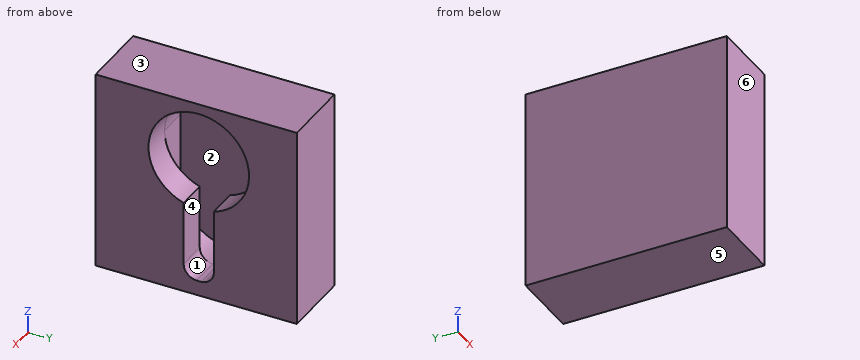
from build123d import *

# Parameters (mm, degrees)
F0_W     = 7
F0_H     = 20
F1_DEPTH = 20
F3_DEPTH = 6
F4_W     = 36.7105286568
F4_H     = 22.0389235765
F5_DEPTH = 3
F6_W     = 20
F6_H     = 20
F7_DEPTH = 3


# Not quite as in the source:
# - after a boolean that leaves OpenCascade's solid faulty, fix() repairs it


with BuildPart() as f1:
    # F0 (on Top) → F1 (new body)
    with BuildSketch(Plane.XY):
        with Locations((-6.9235885665, -0.25)):
            Rectangle(F0_W, F0_H)
    extrude(amount=F1_DEPTH)

    # F2 (on face) → F3 (cut)
    with BuildSketch(Plane.YZ.offset(-3.4235885665)):
        with BuildLine():
            Line((5, 6.5), (5, 14))
            ThreePointArc((5, 14), (0, 19), (-5, 14))
            Line((-5, 14), (-5, 6.5))
            ThreePointArc((-5, 6.5), (-3.5355339059, 2.9644660941), (0, 1.5))
            ThreePointArc((0, 1.5), (3.5355339059, 2.9644660941), (5, 6.5))
        make_face()
    extrude(amount=-F3_DEPTH, mode=Mode.SUBTRACT)

    # F4 (on face) → F5 (cut)
    with BuildSketch(Plane.YZ.offset(-3.4235885665)):
        with Locations((-1.3269511983, 11.0194617882)):
            Rectangle(F4_W, F4_H)
    extrude(amount=-F5_DEPTH, mode=Mode.SUBTRACT)

    # F6 (on face) → F7 (join)
    with BuildSketch(Plane.YZ.offset(-6.4235885665)):
        with Locations((-0.25, 10)):
            Rectangle(F6_W, F6_H)
        with BuildLine():
            ThreePointArc((-1.5, 9.2303039929), (0, 19), (1.5, 9.2303039929))
            Line((1.5, 9.2303039929), (1.5, 2.8392676962))
            ThreePointArc((1.5, 2.8392676962), (1.1297736268, 1.9163028593), (0.2243504639, 1.505035849))
            ThreePointArc((0.2243504639, 1.505035849), (0, 1.5), (-0.2243504639, 1.505035849))
            ThreePointArc((-0.2243504639, 1.505035849), (-1.1297736268, 1.9163028593), (-1.5, 2.8392676962))
            Line((-1.5, 2.8392676962), (-1.5, 9.2303039929))
        make_face(mode=Mode.SUBTRACT)
    extrude(amount=F7_DEPTH)

    add(f1.part.fix(), mode=Mode.REPLACE)


solid = f1.part
Model file for the job. Use its own axes, mm. Face numbers are marked on the shaded views. A direction names the side the tool comes from. Give positions to 0.01 mm unless a question says otherwise; leave off trailing zeros. Loops run counter-clockwise (first coordinate to the right, second up) from the corner with the lowest first, then second, coordinate; pieces in that order, holes last. Notation, with made-up numbers: (-1, -8) - (42, -8) arc R29 cw to (42, 29) - close; hole circle Ø5 at (80, -4). An arc over 180 degrees is marked (long way). Use one line per item in the form item = value.
(1) Pull direction Y, two halves, no side cores. Call the marked faces 4, 5 and 6: pulls with the +Y half, pulls with the -Y half, needs draft (parallel to the pull), parting line crosses it, or undercut.
Determined:
face_4 = undercut
face_5 = needs draft
face_6 = pulls with the -Y half
(2) Drill centre lines: L1, parallel to Z at x = -5.5, y = 0; L2, parallel to Y at x = -4.25, z = 14; L3, parallel to X at y = 2.75, z = 7.75. Where is each one in solid material? Low to high.
Determined:
L1 = 0 to 1.5, 19 to 20
L2 = -10.25 to -5, 5 to 9.75
L3 = -10.42 to -9.42, -6.42 to -3.42
(3) Cut at A-A (z = 8.5). Give the cut face in (x, y), then the cut area to 3 significant figures.
Determined:
outline = (-10.42, -10.25) - (-3.42, -10.25) - (-3.42, -1.5) - (-6.42, -1.5) - (-6.42, -5) - (-9.42, -5) - (-9.42, 5) - (-6.42, 5) - (-6.42, 1.5) - (-3.42, 1.5) - (-3.42, 9.75) - (-10.42, 9.75) - close
area = 101 mm^2
(4) Cut at C-C (y = 2.75). Give the cut face in (x, z), then the cut area to 3 significant figures.
Determined:
outline = (-10.42, 0) - (-3.42, 0) - (-3.42, 9.82) - (-6.42, 9.82) - (-6.42, 2.32) - (-9.42, 2.32) - (-9.42, 18.18) - (-3.42, 18.18) - (-3.42, 20) - (-10.42, 20) - close
area = 67.4 mm^2
(5) 3-axis set-ups, long thin cutter, end or side, ignore diameter. For the marked faces 1, 2 and 3: which of +Z, -Z, +X, -X, +Y, -Y reach the whole face in a straight line?
Determined:
face_1 = +X
face_2 = none
face_3 = +Z, +X, -X, +Y, -Y
(6) Cut at D-D (x = -4.25). Give the cut face in (y, z), then the cut area to 3 significant figures.
Determined:
outline = (-10.25, 0) - (9.75, 0) - (9.75, 20) - (-10.25, 20) - close; hole (-1.5, 2.84) arc R1.34 ccw to (-0.22, 1.51) arc R5 ccw to (0.22, 1.51) arc R1.34 ccw to (1.5, 2.84) - (1.5, 9.23) arc R5 ccw (long way) to (-1.5, 9.23) - close
area = 300 mm^2
(7) Drop a flat-ended pin along its axis: P1, Ø8, axis at y = 0.5, z = 14.5, coming from the +X side. Give the stop position or say it passes through.
Determined:
P1 = -9.42
(8) Cut at B-B (x = -7.5). Give the cut face in (y, z).
Determined:
outline = (-10.25, 0) - (9.75, 0) - (9.75, 20) - (-10.25, 20) - close; hole (-5, 6.5) arc R5 ccw to (5, 6.5) - (5, 14) arc R5 ccw to (-5, 14) - close
